Source: CAD feature listing. Evaluate the final solid. Frame: model axes, mm. Face numbers are marked on the shaded views. A direction names the side the tool comes from. Round coordinates to 2 decimals unless told otherwise and drop trailing zeros. Order: outer loops, then holes, each group sorted by start corner. A loop starts at its lowest first (then second) coordinate and runs counter-clockwise, first axis right, second up. Notation, with made-up numbers: (78, 24) -> (112, 24) arc R25 cw to (112, 60) -> close; hole circle Ø8 at (87, -34.5). An arc over 180 degrees is marked (long way). Write item = value, one per line. Start each with the question number.
(1) Draft query along X for the marked faces 6, 7 and 8. Return one class per face: released by +X, released by -X, zero draft, split by the parting line, or undercut.
(2) Cut plane C-C on y = -2.75. Return the cut outline in (x, z), then the cut area to 3 significant figures.
(3) Ray query, line 1 (Z direction, x = -3.9, y = -5.5); line 2 (Z direction, x = -4.5, y = -1.25); line 3 (Z direction, x = -1.25, y = 6.5). Return the intervals inside material, ascending.
(4) Reachability of the marked faces 1, 2, 3, 4 and 5 from +Z, -Z, +X, -X, +Y, -Y: full face, straight path, thin tool, end or side. Return the list, or none.
(5) Cut plane B-B on z = -3.9. Return the cut outline in (x, y), then the cut area to 3 significant figures.
(6) Cut plane D-D on x = -3.9. Give the number of separate pieces and of enclosed holes in the cut face, then the cut area to 3 significant figures.
(7) Contact query for flat-ended pins moving along their axis: pin 1 Ø2.5 at (y, z) = (4, -11.9) entering from +X; pin 2 Ø0.6 at (x, y) = (-3, -0.5) entering from -Z; pin 3 Ø1.5 at (y, z) = (-4, -39) entering from -X; pin 4 Ø5 at (y, z) = (4, -43.9) entering from +X. Output: stop coordinate, or through.
(8) Cut plane A-A on y = 4. Return the cut outline in (x, z).
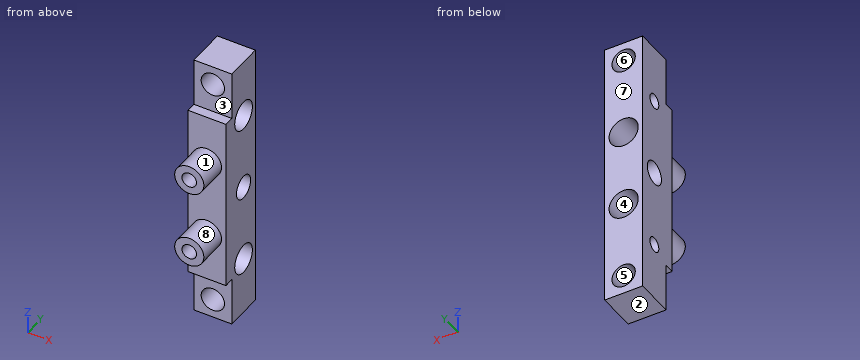
Autodesk Inventor part; units mm, degrees
ref_plane "YZ Plane" through (0, 0, 0) normal (1, 0, 0) x (0, 1, 0)
ref_plane "XZ Plane" through (0, 0, 0) normal (0, 1, 0) x (-1, 0, 0)
ref_plane "XY Plane" through (0, 0, 0) normal (0, 0, 1) x (1, 0, 0)
sketch "Sketch1" plane through (0, 0, 0) normal (0, 1, 0) x (-1, 0, 0)
  line L0 (0, 0) -> (7.8, 0)
  line L1 (7.8, 0) -> (7.8, -55.8)
  line L2 (7.8, -55.8) -> (0, -55.8)
  line L3 (0, -55.8) -> (0, 0)
  line L4 (3.9, 0) -> (3.9, -55.8) construction
  line L5 (7.8, -27.9) -> (0, -27.9) construction
  circle A0 centre (3.9, -19.9) radius 3
  circle A1 centre (3.9, -19.9) radius 1.5
  circle A2 centre (3.9, -35.9) radius 3
  circle A3 centre (3.9, -35.9) radius 1.5
  circle A4 centre (3.9, -3.9) radius 2.4
  circle A5 centre (3.9, -51.9) radius 2.4
  line L6 (0, -9.9) -> (7.8, -9.9)
  line L7 (0, -45.9) -> (7.8, -45.9)
  dimension "d0" = 7.8
  dimension "d1" = 55.8
  dimension "d3" = 6
  dimension "d4" = 3
  dimension "d25" = 8
  dimension "d26" = 4.8
  dimension "d27" = 16
  dimension "d28" = 18
extrude "Extrusion1" add sketch "Sketch1" along normal blind 8 contours L0 L1 L6 L3 | L6 L1 L7 L3 | L7 L1 L2 L3
extrude "Extrusion2" add sketch "Sketch1" against normal blind 2 contours L6 L1 L7 L3 | A0 | A2
extrude "Extrusion3" add sketch "Sketch1" against normal blind 6 from surface at -2 contours A0 | A2
sketch "Sketch2" plane through (0, 8, 0) normal (1, 0, 0) x (0, 0, -1)
  line L0 (0, 0) -> (55.8, 0) construction
  line L1 (0, -8) -> (0, 0) construction
  line L2 (45.9, -10) -> (9.9, -10) construction
  line L3 (55.8, 0) -> (55.8, -10) construction
  line L4 (27.9, 0) -> (27.9, -10) construction
  line L5 (9.9, -10) -> (45.9, -10) construction
  circle A0 centre (27.9, -4) radius 2.4
  line L6 (55.8, 0) -> (0, 0)
  line L7 (11.9, 0) -> (11.9, -10) construction
  circle A1 centre (11.9, -4) radius 1.5
  circle A2 centre (11.9, -4) radius 3
  circle A3 centre (43.9, -4) radius 1.5
  circle A4 centre (43.9, -4) radius 3
  point P0 (0, -10)
  dimension "d11" = 4
  dimension "d12" = 4.8
  dimension "d17" = 4
  dimension "d18" = 3
  dimension "d19" = 6
  dimension "d22" = 16
extrude "Extrusion4" cut sketch "Sketch2" against normal through all contours A0
extrude "Extrusion5" cut sketch "Sketch2" against normal blind 6 contours A1 | A2 | A3 | A4
extrude "Extrusion6" cut sketch "Sketch2" against normal through all contours A1 | A3
properties part number "diff_gear_holder_4"
Evaluation:
q1.face_6 = undercut
q1.face_7 = zero draft
q1.face_8 = split by the parting line
q2.outline = circle Ø6 at (-3.9, -35.9); circle Ø6 at (-3.9, -19.9); hole circle Ø3 at (-3.9, -35.9); hole circle Ø3 at (-3.9, -19.9)
q2.area = 42.4 mm^2
q3.line_1 = -38.9 to -37.4, -34.4 to -32.9, -22.9 to -21.4, -18.4 to -16.9
q3.line_2 = -45.9 to -37.27, -34.53 to -21.27, -18.53 to -9.9
q3.line_3 = -55.8 to -45.56, -42.24 to -37.31, -34.49 to -21.31, -18.49 to -13.56, -10.24 to 0
q4.face_1 = -Y
q4.face_2 = -Z, +X, -X, +Y, -Y
q4.face_3 = +Z, +X, -X, -Y
q4.face_4 = +Y
q4.face_5 = +Y, -Y
q5.outline = (-7.8, 0) -> (-6.3, 0) -> (-6.3, 8) -> (-7.8, 8) -> close; (-1.5, 0) -> (0, 0) -> (0, 8) -> (-1.5, 8) -> close
q5.area = 24.0 mm^2
q6.separate_pieces = 5
q6.enclosed_holes = 3
q6.area = 295 mm^2
q7.pin_1 = through
q7.pin_2 = -45.9
q7.pin_3 = -5.76
q7.pin_4 = -6
q8.outline = (-7.8, -55.8) -> (0, -55.8) -> (0, -46.9) -> (-6, -46.9) -> (-6, -45.4) -> (-7.8, -45.4) -> close; (-7.8, -42.4) -> (-6, -42.4) -> (-6, -40.9) -> (0, -40.9) -> (0, -30.3) -> (-7.8, -30.3) -> close; (-7.8, -25.5) -> (0, -25.5) -> (0, -14.9) -> (-6, -14.9) -> (-6, -13.4) -> (-7.8, -13.4) -> close; (-7.8, -10.4) -> (-6, -10.4) -> (-6, -8.9) -> (0, -8.9) -> (0, 0) -> (-7.8, 0) -> close; hole circle Ø6 at (-3.9, -35.9); hole circle Ø6 at (-3.9, -19.9); hole circle Ø4.8 at (-3.9, -51.9); hole circle Ø4.8 at (-3.9, -3.9)
